from build123d import *

# Parameters (mm, degrees)
EXTRUDE_THIN1_DEPTH = 2.6
BOSS_EXTRUDE1_DEPTH = 3
EXTRUDE_THIN2_DEPTH = 5.6
SKETCH5_R           = 1.75
CUT_EXTRUDE1_DEPTH  = 31.537946797
FILLET1_R           = 10


# Read off the part's stored shape, not the designer's step: Extrude-Thin1
with BuildPart() as part:
    # Extrude-Thin1 outline → Extrude-Thin1 (new body)
    with BuildSketch(Plane(origin=(0, 0, 0), x_dir=(1, 0, 0), z_dir=(0, 1, 0))):
        with BuildLine():
            ThreePointArc((5.101086932, 18.009411765), (0, 22.2), (-5.101086932, 18.009411765))
            Line((-5.101086932, 18.009411765), (-8.338315178, 1.65))
            ThreePointArc((-8.338315178, 1.65), (0, -8.5), (8.338315178, 1.65))
            Line((8.338315178, 1.65), (5.101086932, 18.009411765))
        make_face()
        with BuildLine():
            Line((-5.885869537, 1.164705882), (-2.648641292, 17.524117647))
            ThreePointArc((-2.648641292, 17.524117647), (0, 19.7), (2.648641292, 17.524117647))
            Line((2.648641292, 17.524117647), (5.885869537, 1.164705882))
            ThreePointArc((5.885869537, 1.164705882), (0, -6), (-5.885869537, 1.164705882))
        make_face(mode=Mode.SUBTRACT)
    extrude(amount=EXTRUDE_THIN1_DEPTH)

    # Sketch2 → Boss-Extrude1 (add)
    # profile 1 of 2: a face of its own
    with BuildSketch(Plane(origin=(0, 2.6, 0), x_dir=(1, 0, 0), z_dir=(0, 1, 0))):
        with BuildLine():
            Line((8.338315178, 1.65), (5.101086932, 18.009411765))
            ThreePointArc((5.101086932, 18.009411765), (0, 22.2), (-5.101086932, 18.009411765))
            Line((-5.101086932, 18.009411765), (-8.338315178, 1.65))
            ThreePointArc((-8.338315178, 1.65), (0, -8.5), (8.338315178, 1.65))
        make_face()
        with BuildLine():
            ThreePointArc((5.885869537, 1.164705882), (0, -6), (-5.885869537, 1.164705882))
            Line((-5.885869537, 1.164705882), (-2.648641292, 17.524117647))
            ThreePointArc((-2.648641292, 17.524117647), (0, 19.7), (2.648641292, 17.524117647))
            Line((2.648641292, 17.524117647), (5.885869537, 1.164705882))
        make_face(mode=Mode.SUBTRACT)
    # profile 2 of 2: a face of its own
    with BuildSketch(Plane(origin=(0, 2.6, 0), x_dir=(1, 0, 0), z_dir=(0, 1, 0))):
        with BuildLine():
            Line((-5.885869537, 1.164705882), (-2.648641292, 17.524117647))
            ThreePointArc((-2.648641292, 17.524117647), (0, 19.7), (2.648641292, 17.524117647))
            Line((2.648641292, 17.524117647), (5.885869537, 1.164705882))
            ThreePointArc((5.885869537, 1.164705882), (0, -6), (-5.885869537, 1.164705882))
        make_face()
    extrude(amount=BOSS_EXTRUDE1_DEPTH)

    # Sketch4 → Extrude-Thin2 (add, through all)
    with BuildSketch(Plane(origin=(0, 5.6, 0), x_dir=(1, 0, 0), z_dir=(0, 1, 0))):
        with BuildLine():
            Line((10.796856578, -1.499295844), (18.15807251, -5.749295844))
            ThreePointArc((18.15807251, -5.749295844), (19.658776666, -11.35), (14.05807251, -12.850704156))
            Line((14.05807251, -12.850704156), (6.696856578, -8.600704156))
            ThreePointArc((6.696856578, -8.600704156), (5.196152423, -3), (10.796856578, -1.499295844))
        make_face()
        with BuildLine():
            Line((9.546856578, -3.664359354), (16.90807251, -7.914359354))
            ThreePointArc((16.90807251, -7.914359354), (17.493713156, -10.1), (15.30807251, -10.685640646))
            Line((15.30807251, -10.685640646), (7.946856578, -6.435640646))
            ThreePointArc((7.946856578, -6.435640646), (7.361215932, -4.25), (9.546856578, -3.664359354))
        make_face(mode=Mode.SUBTRACT)
    extrude(amount=-EXTRUDE_THIN2_DEPTH)

    # Sketch5 → Cut-Extrude1 (cut, through all)
    with BuildSketch(Plane(origin=(0, 5.6, 0), x_dir=(1, 0, 0), z_dir=(0, 1, 0))):
        with Locations(Location((0, 0, 0), (0, 0, 270))):
            Circle(SKETCH5_R)
    extrude(amount=-CUT_EXTRUDE1_DEPTH, mode=Mode.SUBTRACT)

    # Fillet1
    # the kernel refuses this fillet: 10 mm, written as the material it adds along each edge
    with BuildSketch(Plane(origin=(5.055074156, 5.6, 6.833463637), x_dir=(0.7701817690160239, 0, 0.6378244607063513), z_dir=(0, -1, 0))) as fillet1_piece_1_section:
        with BuildLine():
            CenterArc((5.914673675, 9.859092079), FILLET1_R, 220.025396245, 40.344818113)
            Line((-1.74292086, 3.427821136), (-2.508680314, 2.784694042))
            ThreePointArc((-2.508680314, 2.784694042), (-1.566456977, 1.360530409), (-0.970808966, -0.239854019))
            Line((-0.970808966, -0.239854019), (0.416050435, -0.909341539))
            ThreePointArc((0.416050435, -0.909341539), (2.224378819, -0.671981767), (4.074579357, -0.985909208))
            Line((4.074579357, -0.985909208), (4.241860659, 0))
        make_face()
    fillet1_piece_1 = extrude(amount=13.604651647, mode=Mode.PRIVATE)
    fillet1_piece_1 = split(fillet1_piece_1, bisect_by=Plane(origin=(5.032331635, 0, 8.326315452), z_dir=(0, 1, 0)), keep=Keep.TOP, mode=Mode.PRIVATE)
    add(fillet1_piece_1)
    with BuildSketch(Plane(origin=(8.445490183, 5.6, 0.961090818), x_dir=(0.9339582285833896, 0, 0.35738218654736686), z_dir=(0, -1, 0))) as fillet1_piece_2_section:
        with BuildLine():
            CenterArc((6.080721922, -9.875226453), FILLET1_R, 99.060486088, 48.806816394)
            Line((-2.38746333, -4.556407174), (-3.234281856, -4.024525246))
            ThreePointArc((-3.234281856, -4.024525246), (-1.88007285, -1.868465389), (-0.968377858, 0.249488126))
            Line((-0.968377858, 0.249488126), (0.425065104, 0.905162779))
            ThreePointArc((0.425065104, 0.905162779), (2.23094582, 0.649847195), (4.348474242, 0.987522645))
            Line((4.348474242, 0.987522645), (4.505951304, 0))
        make_face()
    fillet1_piece_2 = extrude(amount=15.860022231, mode=Mode.PRIVATE)
    fillet1_piece_2 = split(fillet1_piece_2, bisect_by=Plane(origin=(9.506243906, 0, -0.256428974), z_dir=(0, 1, 0)), keep=Keep.TOP, mode=Mode.PRIVATE)
    add(fillet1_piece_2)


solid = part.part
CAD build for the part. Positions are in the model's coordinates, mm. A direction names the side the tool comes from. Coordinates: 2 decimals unless noted, no trailing zeros. Write each loop counter-clockwise with the first axis right and the second up, starting at its lowest first coordinate (ties: lowest second). Pieces come first, ordered by that corner, then holes. Notation, with made-up numbers: M -18.5,-18.75 L 1.5,-18.75 A27 ccw 1.5,14.25 Z; hole C 28,45.5 d2. An arc over 180 degrees is marked long. Return JSON: item names as keys, results as strings.
Item 1: Slice it at C-C, the plane y = 5. Write the cut outline in (x, z).
Findings below:
{"outline": "M -8.34,-1.65 L -5.1,-18.01 A5.2 ccw 5.1,-18.01 L 7.84,-4.15 A10 cw 12.65,2.57 L 18.16,5.75 A4.1 ccw 14.06,12.85 L 8.32,9.54 A10 cw 1.53,8.36 A8.5 ccw Z; hole C 0,0 d3.5; hole M 7.95,6.44 A1.6 ccw 9.55,3.66 L 16.91,7.91 A1.6 ccw 15.31,10.69 Z"}
Item 2: Slice it at B-B, the plane z = 5.05. Write the cut outline in (x, y).
Findings below:
{"outline": "M -6.84,0 L -3.24,0 L -3.24,2.6 L 3.24,2.6 L 3.24,0 L 7.15,0 L 7.15,5.6 L -6.84,5.6 Z; M 11.95,0 L 16.95,0 L 16.95,5.6 L 11.95,5.6 Z"}
Item 3: Slice it at A-A, the plane x = 0. Write the cut outline in (y, z).
Findings below:
{"outline": "M 0,-22.2 L 5.6,-22.2 L 5.6,-1.75 L 2.6,-1.75 L 2.6,-19.7 L 0,-19.7 Z; M 0,6 L 2.6,6 L 2.6,1.75 L 5.6,1.75 L 5.6,8.5 L 0,8.5 Z"}
Item 4: Two-plate mould, pull along X, no slides. Class faces 4 (the cylindrical face through (0.1, 2.8, -22.2)), 5 (the flat face through (-6.697, 2.761, -9.944)), 6 (the flat face through (4.245, 1.282, -9.459)): +X half, -X half, draft (parallel to the pull), parting line (faces both ways), or undercut.
Findings below:
{"face 4": "parting line", "face 5": "-X half", "face 6": "undercut"}
Item 5: Probe line 1 (Y direction, x = -1.5, z = 3.5); line 2 (Z direction, x = 16, y = 3.85); line 3 (X direction, y = 1.8, z = -5). List the from-to ranges inside material, lowest first. Write a range as from..to.
Findings below:
{"line 1": "y = 2.6..5.6", "line 2": "z = 4.5..7.39, 10.9..13.4", "line 3": "x = -7.68..-5.13, 5.13..7.68"}
Item 6: Slice it at D-D, the plane z = -16. Write the cut outline in (x, y), and give its area (3 significant figures).
Findings below:
{"outline": "M -5.5,0 L -2.95,0 L -2.95,2.6 L 2.95,2.6 L 2.95,0 L 5.5,0 L 5.5,5.6 L -5.5,5.6 Z", "area": "46.2 mm2"}
Item 7: Drop flat-ended pins along their axis: pin 1 Ø1.5 at (y, z) = (1, 5) entering from -X; pin 2 Ø3 at (y, z) = (1.5, 8.5) entering from +X; pin 3 Ø1 at (x, y) = (10, 0.5) entering from +Z; pin 4 Ø2 at (y, z) = (2, -12) entering from -X. Give the stop position or say it passes through.
Findings below:
{"pin 1": "stops at x = -7.36", "pin 2": "stops at x = 20.21", "pin 3": "stops at z = 10.8", "pin 4": "stops at x = -6.49"}
Item 8: Which spindle directions (+Z, -Z, +X, -X, +Y, -Y) get a long thin tool onto all of the face, cutting with end or side? Do faces 1 (the flat face through (11.68, 2.84, 8.59)), 2 (the cylindrical face through (0, 1, 6)), 3 (the flat face through (15.37, 2.84, 4.14)). Say none if no direction does.
Findings below:
{"face 1": "+Y, -Y", "face 2": "-Y", "face 3": "-Z, +X, +Y, -Y"}
